Work out the finished part from the listing and answer in its coordinate system (mm). Face numbers are marked on the shaded views. A direction names the side the tool comes from. Coordinates: 2 decimals unless noted, no trailing zeros. Loops run counter-clockwise (first coordinate to the right, second up) from the corner with the lowest first, then second, coordinate; pieces in that order, holes last. Notation, with made-up numbers: (46.25, -13.5) -> (99.25, -13.5) arc R27 ccw to (99.25, 17.5) -> close; hole circle Ø5 at (-21.5, 12.5). An arc over 180 degrees is marked (long way). Answer as CSV lines item,"result".
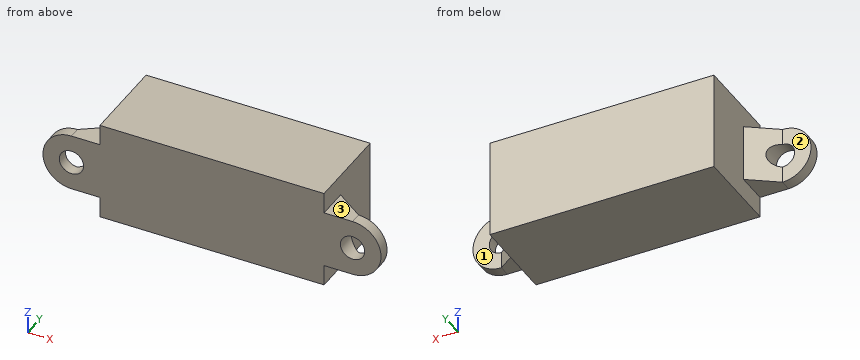
```python
from build123d import *

# Parameters (mm, degrees)
CROQUIS1_R                 = 1.6
SALIENTE_EXTRUIR2_DEPTH    = 11.5
CORTAR_EXTRUIR1_DEPTH      = 26.875905781
CORTAR_EXTRUIR1_DEPTH_BACK = 26.875905781


with BuildPart() as part:
    # Croquis1 → Saliente-Extruir2 (new body)
    with BuildSketch(Plane(origin=(0, 0, 0), x_dir=(1, 0, 0), z_dir=(0, 1, 0))):
        with BuildLine():
            Line((-14.75, -6.5), (14.75, -6.5))
            Line((14.75, -6.5), (14.75, -3.75))
            Line((14.75, -3.75), (18.5, -3.75))
            ThreePointArc((18.5, -3.75), (22.25, 0), (18.5, 3.75))
            Line((18.5, 3.75), (14.75, 3.75))
            Line((14.75, 3.75), (14.75, 6.5))
            Line((14.75, 6.5), (-14.75, 6.5))
            Line((-14.75, 6.5), (-14.75, 3.75))
            Line((-14.75, 3.75), (-18.5, 3.75))
            ThreePointArc((-18.5, 3.75), (-22.25, 0), (-18.5, -3.75))
            Line((-18.5, -3.75), (-14.75, -3.75))
            Line((-14.75, -3.75), (-14.75, -6.5))
        make_face()
        with Locations(Location((-18.5, 0, 0), (0, 0, 270))):
            Circle(CROQUIS1_R, mode=Mode.SUBTRACT)
        with Locations(Location((18.5, 0, 0), (0, 0, 90))):
            Circle(CROQUIS1_R, mode=Mode.SUBTRACT)
    extrude(amount=SALIENTE_EXTRUIR2_DEPTH)

    # Croquis2 → Cortar-Extruir1 (cut, two sides: drawn at the far end of the back side and taken through both)
    with BuildSketch(Plane.XY.offset(-CORTAR_EXTRUIR1_DEPTH_BACK)):
        Polygon((22.25, 11.5), (22.25, 1.5), (18.5, 1.5), (14.75, 4.125778268), (14.75, 11.5), align=None)
        Polygon((-22.25, 11.5), (-22.25, 1.5), (-18.5, 1.5), (-14.75, 4.125778268), (-14.75, 11.5), align=None)
    extrude(amount=CORTAR_EXTRUIR1_DEPTH + CORTAR_EXTRUIR1_DEPTH_BACK, mode=Mode.SUBTRACT)


solid = part.part
```
(1) A cutting plane is placed at D-D, the plane z = -2.5. Write down the section's boundary in (x, y).
Computed values:
outline,"(-21.3, 0) -> (21.3, 0) -> (21.3, 1.5) -> (18.5, 1.5) -> (14.75, 4.13) -> (14.75, 11.5) -> (-14.75, 11.5) -> (-14.75, 4.13) -> (-18.5, 1.5) -> (-21.3, 1.5) -> close"
(2) Consider line 1 along X through (y, z) = (1.4, 0); line 2 along Z through (x, y) = (-18.5, 0.85). Determine where each line is inside the solid, lowest interval first.
Computed values:
line 1,"-22.25 to -20.1, -16.9 to 16.9, 20.1 to 22.25"
line 2,"-3.75 to -1.6, 1.6 to 3.75"
(3) Flat-ended cylindrical pins translate along their axes: pin 1 Ø5 at (x, z) = (-18.5, 0) entering from -Y; pin 2 Ø3.5 at (y, z) = (7, 2.5) entering from +X; pin 3 Ø3 at (x, y) = (-16.5, 2) entering from +Z; pin 4 Ø2.5 at (x, z) = (18.5, 0) entering from +Y (3 decimals). Find the tip coordinate at first contact, or state that the pin passes through.
Computed values:
pin 1,"y = 0"
pin 2,"x = 14.75"
pin 3,"z = 3.75"
pin 4,"through"
(4) A cutting plane is placed at C-C, the plane x = 15.5. Write down the section's boundary in (y, z).
Computed values:
outline,"(0, -3.75) -> (3.6, -3.75) -> (3.6, 3.75) -> (0, 3.75) -> close"
(5) A cutting plane is placed at A-A, the plane z = 0. Write down the section's boundary in (x, y), and give its area (3 significant figures).
Computed values:
outline,"(-22.25, 0) -> (-20.1, 0) -> (-20.1, 1.5) -> (-22.25, 1.5) -> close; (-16.9, 0) -> (16.9, 0) -> (16.9, 2.62) -> (14.75, 4.13) -> (14.75, 11.5) -> (-14.75, 11.5) -> (-14.75, 4.13) -> (-16.9, 2.62) -> close; (20.1, 0) -> (22.25, 0) -> (22.25, 1.5) -> (20.1, 1.5) -> close"
area,"360 mm2"
(6) A cutting plane is placed at B-B, the plane y = 2. Write down the section's boundary in (x, z), and give its area (3 significant figures).
Computed values:
outline,"(-17.79, -3.75) -> (-14.75, -3.75) -> (-14.75, -6.5) -> (14.75, -6.5) -> (14.75, -3.75) -> (17.79, -3.75) -> (17.79, -1.43) arc R1.6 cw to (17.79, 1.43) -> (17.79, 3.75) -> (14.75, 3.75) -> (14.75, 6.5) -> (-14.75, 6.5) -> (-14.75, 3.75) -> (-17.79, 3.75) -> (-17.79, 1.43) arc R1.6 cw to (-17.79, -1.43) -> close"
area,"425 mm2"
(7) Which of the six approach directions +Z, -Z, +X, -X, +Y, -Y give full straight-line access (tool end or side, diameter ignored) to the marked faces 1, 2 and 3?
Computed values:
face 1,"+Z, -Z, +X, +Y"
face 2,"+Z, -Z, -X, +Y"
face 3,"+Z, +X, +Y, -Y"
